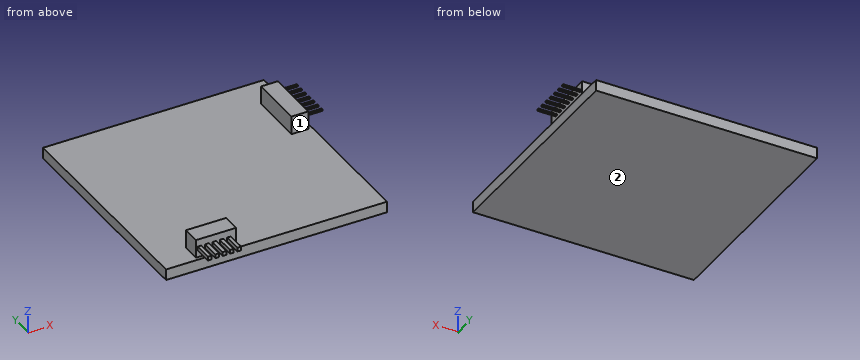
```python
from build123d import *

# Parameters (mm, degrees)
SKETCH2_W           = 60
SKETCH2_H           = 60
BOSS_EXTRUDE1_DEPTH = 3
SKETCH3_W           = 10.924948593
SKETCH3_H           = 4.874207834
SKETCH3_W_2         = 4.538055569
SKETCH3_H_2         = 14.86497051
BOSS_EXTRUDE2_DEPTH = 5
SKETCH4_W           = 1.00253682
SKETCH4_H           = 1.076798806
BOSS_EXTRUDE3_DEPTH = 5
LPATTERN1_COUNT     = 5
LPATTERN1_PITCH     = 2
SKETCH5_W           = 0.358984387
SKETCH5_H           = 0.512834838
BOSS_EXTRUDE4_DEPTH = 5
LPATTERN2_COUNT     = 7
LPATTERN2_PITCH     = 2


with BuildPart() as part:
    # Sketch2 → Boss-Extrude1 (new body)
    with BuildSketch(Plane.XY):
        with Locations((0.566037736, -6.438679245)):
            Rectangle(SKETCH2_W, SKETCH2_H)
    extrude(amount=BOSS_EXTRUDE1_DEPTH)

    # Sketch3 → Boss-Extrude2 (add)
    with BuildSketch(Plane.XY.offset(3)):
        with Locations((-15.317156757, -33.036727165)):
            Rectangle(SKETCH3_W, SKETCH3_H)
        with Locations((27.206104689, 7.432485255)):
            Rectangle(SKETCH3_W_2, SKETCH3_H_2)
    extrude(amount=BOSS_EXTRUDE2_DEPTH)

    # Sketch4 → Boss-Extrude3 (add)
    with BuildSketch(Plane.XZ.offset(35.473831082)):
        with Locations((-19.804086394, 5.472695433)):
            Rectangle(SKETCH4_W, SKETCH4_H)
    boss_extrude3 = extrude(amount=BOSS_EXTRUDE3_DEPTH)

    # LPattern1: Boss-Extrude3 ×5
    with Locations(*[(i * LPATTERN1_PITCH, 0, 0) for i in range(1, LPATTERN1_COUNT)]):
        add(boss_extrude3)

    # Sketch5 → Boss-Extrude4 (add)
    with BuildSketch(Plane(origin=(29.475132473, 0, 0), x_dir=(0, 0, -1), z_dir=(1, 0, 0))):
        with Locations((-5.618353943, 14.22099245)):
            Rectangle(SKETCH5_W, SKETCH5_H)
    boss_extrude4 = extrude(amount=BOSS_EXTRUDE4_DEPTH)

    # LPattern2: Boss-Extrude4 ×7
    with Locations(*[(0, -i * LPATTERN2_PITCH, 0) for i in range(1, LPATTERN2_COUNT)]):
        add(boss_extrude4)


solid = part.part
```
CAD build for the part. Positions are in the model's coordinates, mm. Face numbers are marked on the shaded views. A direction names the side the tool comes from. Round coordinates to 2 decimals unless told otherwise and drop trailing zeros. Order: outer loops, then holes, each group sorted by start corner. A loop starts at its lowest first (then second) coordinate and runs counter-clockwise, first axis right, second up. Notation, with made-up numbers: (7.5, -32) - (15.5, -32) arc R28 ccw to (15.5, 5) - close; hole circle Ø7 at (64.25, 75.5). An arc over 180 degrees is marked (long way). Answer in a Markdown table with one row per item. Add a question column.
(1) Drop flat-ended pins along their axis: pin 1 Ø1.5 at (y, z) = (5.5, 6.5) entering from +X; pin 2 Ø10 at (x, y) = (-16.5, -11.5) entering from +Z; pin 3 Ø2.5 at (y, z) = (-33, 6) entering from -X. Give the stop position or say it passes through.
(2) Band-saw the part on B-B on x = 4.5. List the corners of the cut face in (y, z), and give its area (3 significant figures).
(3) Band-saw the part on C-C on z = 1.25. List the corners of the cut face in (x, y), and give its area (3 significant figures).
(4) Band-saw the part on A-A on y = -33.5. List the corners of the cut face in (x, z), and give its area (3 significant figures).
(5) 3-axis set-ups, long thin cutter, end or side, ignore diameter. For the marked faces 1 and 2: which of +Z, -Z, +X, -X, +Y, -Y reach the whole face in a straight line?
(6) Probe L1, parallel to Y at x = 17.5, z = 0.5; L2, parallel to Y at x = -13.5, z = 5; L3, parallel to Z at x = -21, y = -18. List the from-to ranges inside material, lowest first. Write a range as [from, to].
Data:
| question | item | result |
|---|---|---|
| 1 | pin 1 | stops at x = 29.48 |
| 1 | pin 2 | stops at z = 3 |
| 1 | pin 3 | stops at x = -20.78 |
| 2 | outline | (-36.44, 0) - (23.56, 0) - (23.56, 3) - (-36.44, 3) - close |
| 2 | area | 180 mm^2 |
| 3 | outline | (-29.43, -36.44) - (30.57, -36.44) - (30.57, 23.56) - (-29.43, 23.56) - close |
| 3 | area | 3,600 mm^2 |
| 4 | outline | (-29.43, 0) - (30.57, 0) - (30.57, 3) - (-9.85, 3) - (-9.85, 8) - (-20.78, 8) - (-20.78, 3) - (-29.43, 3) - close |
| 4 | area | 235 mm^2 |
| 5 | face 1 | +Z, +X, -X, -Y |
| 5 | face 2 | -Z, +X, -X, +Y, -Y |
| 6 | L1 | y = [-36.44, 23.56] |
| 6 | L2 | y = [-40.47, -30.6] |
| 6 | L3 | z = [0, 3] |
